Input: part model. Units: mm. Frame: model coordinates. A direction names the side the tool comes from. Round coordinates to 2 decimals unless told otherwise and drop trailing zeros. Loops run counter-clockwise (first coordinate to the right, second up) from the corner with the lowest first, then second, coordinate; pieces in that order, holes last.
(1) Cut plane C-C, the plane y = 4.25. Output: boundary loops of the cut face in (x, z).
(2) First-contact query: pin 1 Ø1.3 at (y, z) = (4, 5) entering from -X; pin 2 Ø0.6 at (y, z) = (4, 4.5) entering from +X; pin 3 Ø2 at (x, z) = (0.5, 0.5) entering from +Y; pin 4 Ø1.4 at (x, y) = (-4, 7.5) entering from -Z. Flat tips, straight axial feed; report the tip coordinate or a pass-through.
(3) Cut plane B-B, the plane x = 3. Output: boundary loops of the cut face in (y, z), and give its area (3 significant figures).
(4) Cut plane A-A, the plane z = 1. Output: boundary loops of the cut face in (x, y), and give its area (3 significant figures).
(5) Access query for faces 1 (the face through (0, 0, 4)), 2 (the face through (-4, 5, 6.3)), 3 (the face through (1.501, 5.07, 6.015)). Directions: +Z, -Z, +X, -X, +Y, -Y. A direction counts if a zero-diameter tool reaches every point of the face in a straight line with its end or side. Return the directions, or none.
(6) Line query: line 1 (X direction, y = 7.25, z = 0); line 2 (Z direction, x = -2.25, y = 1.75); line 3 (Z direction, x = 4, y = 3.5). Output: solid intervals per line, ascending.
(7) Draft query along X for faces 4 (the face through (2.4, 4.93, -2.08)), 5 (the face through (4, 5, 6.3)), 6 (the face through (5.6, 4.9, 6.9)), 7 (the face through (-1.501, 5.07, 6.015)). Return one class per face: released by +X, released by -X, zero draft, split by the parting line, or undercut.
from build123d import *

# Parameters (mm, degrees)
BOSS_EXTRUDE1_DEPTH = 10
FILLET1_R           = 1


with BuildPart() as part:
    # Sketch1 → Boss-Extrude1 (new body)
    with BuildSketch(Plane(origin=(0, 0, 0), x_dir=(1, 0, 0), z_dir=(0, 1, 0))):
        with BuildLine():
            Line((0, -2.5), (0, -7.5))
            Line((0, -7.5), (-5, -7.5))
            ThreePointArc((-5, -7.5), (-5.6, -6.9), (-5, -6.3))
            Line((-5, -6.3), (-1.2, -6.3))
            Line((-1.2, -6.3), (-1.2, -3.5))
            ThreePointArc((-1.2, -3.5), (-3.464834252, -1.298046071), (-3.204293994, 1.85))
            ThreePointArc((-3.204293994, 1.85), (-2.384678752, 2.069615242), (-2.165063509, 1.25))
            ThreePointArc((-2.165063509, 1.25), (-2.165063509, -1.25), (0, -2.5))
        make_face()
    extrude(amount=BOSS_EXTRUDE1_DEPTH)

    # Fillet1
    fillet1_edges = [part.edges().sort_by_distance(p)[0] for p in [
        (-1.2, 5, 6.3),
        (-1.2, 5, 3.5),
    ]]
    fillet(fillet1_edges, radius=FILLET1_R)

    # Mirror1: part across plane


with BuildPart() as part_1:
    add(part.part)
    add(part.part.mirror(Plane(origin=(0, 10, 2.5), x_dir=(0, 0, 1), z_dir=(-1, 0, 0))))


solid = part_1.part
Reported:
1. outline: (-5, 6.3) - (-2.2, 6.3) arc R1 cw to (-1.2, 5.3) - (-1.2, 4.15) arc R1 cw to (-1.73, 3.27) arc R3.7 ccw to (-3.2, -1.85) arc R0.6 ccw to (-2.17, -1.25) arc R2.5 cw (long way) to (2.17, -1.25) arc R0.6 ccw to (3.2, -1.85) arc R3.7 ccw to (1.73, 3.27) arc R1 cw to (1.2, 4.15) - (1.2, 5.3) arc R1 cw to (2.2, 6.3) - (5, 6.3) arc R0.6 ccw to (5, 7.5) - (-5, 7.5) arc R0.6 ccw to start
2. pin 1: stops at x = -1.26
2. pin 2: stops at x = 1.2
2. pin 3: passes through
2. pin 4: stops at z = -1.67
3. outline: (0, -2.06) - (10, -2.06) - (10, 2.17) - (0, 2.17) - close; (0, 6.3) - (10, 6.3) - (10, 7.5) - (0, 7.5) - close
3. area: 54.3 mm2
4. outline: (-3.56, 0) - (-2.29, 0) - (-2.29, 10) - (-3.56, 10) - close; (2.29, 0) - (3.56, 0) - (3.56, 10) - (2.29, 10) - close
4. area: 25.4 mm2
5. face 1: +Z, -Z, +X, -X, -Y
5. face 2: -X, +Y, -Y
5. face 3: +X, +Y, -Y
6. line 1: x = -3.7 to -2.5, 2.5 to 3.7
6. line 2: z = -1.96 to -1.09, 1.09 to 2.94, 6.3 to 7.5
6. line 3: z = 6.3 to 7.5
7. face 4: undercut
7. face 5: zero draft
7. face 6: released by +X
7. face 7: released by -X
